Drawing for the job (mm, zero at the part's lowest x, y, z). Give positions to 0.01 mm unless a question says otherwise; leave off trailing zeros. Order: outer loops, then holes, each group sorted by start corner. A loop starts at its lowest first (then second) coordinate and runs counter-clockwise, first axis right, second up. Notation, with made-up numbers: (13.5, -37) - (47.5, -37) arc R13 cw to (47.5, -29) - close; hole circle Ø10 at (-25, -33.75). An arc over 180 degrees is marked (long way). One line per item, written item: value.
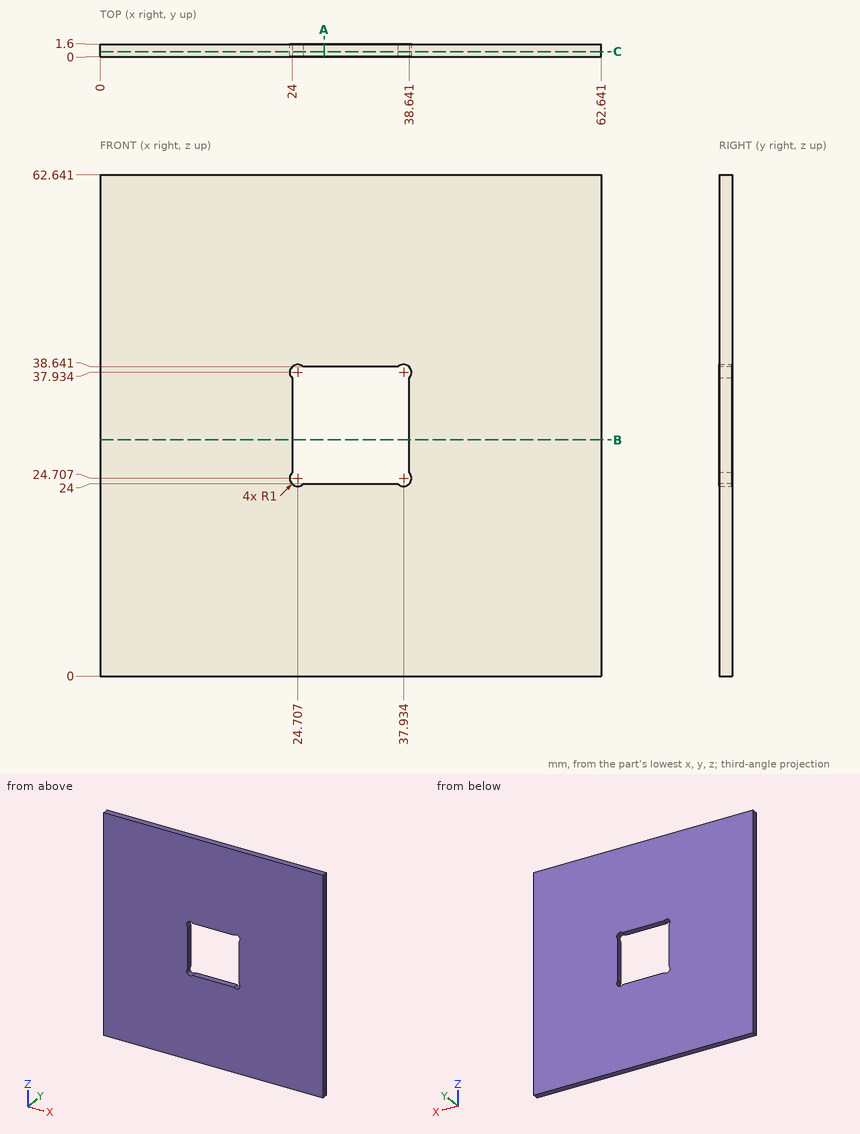
1) Cut at A-A, the plane x = 28. Give the cut face in (y, z), then the cut area to 3 significant figures.
Outcome:
outline: (0, 0) - (1.6, 0) - (1.6, 24) - (0, 24) - close; (0, 38.64) - (1.6, 38.64) - (1.6, 62.64) - (0, 62.64) - close
area: 76.8 mm^2
2) Pin check, flat tip, straight feed: pin 1 (0.5 mm diameter, centred on y = 0.5, z = 33, fed in from -X). Stop position of the tip, or through.
Outcome:
pin 1: stops at x = 0
3) Drill centre lines: line 1 along X through (y, z) = (1.45, 26); line 2 along Z through (x, y) = (25, 1.4). Where is each one in solid material? Low to high. Write a range as from..to.
Outcome:
line 1: x = 0..24, 38.64..62.64
line 2: z = 0..23.75, 38.89..62.64
4) Cut at B-B, the plane z = 29.5. Give the cut face in (x, y), then the cut area to 3 significant figures.
Outcome:
outline: (0, 0) - (24, 0) - (24, 1.6) - (0, 1.6) - close; (38.64, 0) - (62.64, 0) - (62.64, 1.6) - (38.64, 1.6) - close
area: 76.8 mm^2
5) Cut at C-C, the plane y = 0.65. Give the cut face in (x, z).
Outcome:
outline: (0, 0) - (62.64, 0) - (62.64, 62.64) - (0, 62.64) - close; hole (24, 25.41) arc R1 ccw to (25.41, 24) - (37.23, 24) arc R1 ccw to (38.64, 25.41) - (38.64, 37.23) arc R1 ccw to (37.23, 38.64) - (25.41, 38.64) arc R1 ccw to (24, 37.23) - close
